Autodesk Fusion 360 part; units mm, degrees
sketch "Esquisse1" plane through (0, 0, 0) normal (0, 0, 1) x (1, 0, 0)
  circle A0 centre (0, 0) radius 12.5
  line L0 (-5.3, -5.3) -> (5.3, -5.3)
  line L1 (5.3, -5.3) -> (5.3, 5.3)
  line L2 (5.3, 5.3) -> (-5.3, 5.3)
  line L3 (-5.3, 5.3) -> (-5.3, -5.3)
  dimension "d1" = 25
  dimension "d4" = 10.6
  dimension "d5" = 5.3
  dimension "d6" = 5.3
extrude "Extrusion1" add sketch "Esquisse1" along normal blind 22 contours A0 | L0 L1 L2 L3
extrude "Extrusion2" cut sketch "Esquisse1" along normal blind 6 contours L0 L1 L2 L3
sketch "Esquisse2" plane through (0, 0, 22) normal (0, 0, 1) x (-1, 0, 0)
  circle A0 centre (0, 0) radius 12.5
  circle A1 centre (0, 0) radius 1.5
  dimension "d9" = 3
extrude "Extrusion3" cut sketch "Esquisse2" against normal blind 22 contours A1
hole "Perçage2" at (0, 0, 6) direction (0, 0, 1) diameter 8 depth 10 tip angle 180
fillet "Congé1" radius 10 1 edges at (-11.6541, -4.5202, 22)
chamfer "Chanfrein1" distance 0.5 angle 45 4 edges at (-5.3, 0, 0) (0, -5.3, 0) (5.3, 0, 0) (0, 5.3, 0)
equation "d5 = d4 / 2"
equation "d6 = d5"
Could you check a few things on this model? Use its own coordinates, in mm. A direction names the side the tool comes from. Coordinates: 2 decimals unless noted, no trailing zeros. Loops run counter-clockwise (first coordinate to the right, second up) from the corner with the lowest first, then second, coordinate; pieces in that order, holes last.
1. Imagine slicing it at B-B (z = 10.25). Please give me the cut outline in (x, y), and give its area (3 significant figures).
2. Imagine slicing it at A-A (z = 2.25). Please give me the cut outline in (x, y).
3. We'd pull the mould along X, two halves only. Please class faces 1 (the face through (0, -8, 0)), 2 (the face through (0, -5.3, 3)), 3 (the face through (11.923, -3.755, 5.916)): released by +X, released by -X, zero draft, split by the parting line, or undercut.
4. For P1, Ø6, axis at y = -6.5, z = 12, coming from the +X side; P2, Ø4, axis at x = -2, y = 3.5, coming from the +Z side; P3, Ø6, axis at x = 2, z = 19.5, coming from the -Y side; P4, Ø4, axis at x = 0, y = 0, coming from the -Z side, each with a flat end and sliding along its axis, tell me the tip position at first contact or that it passes through.
5. I need wall thicknesses on L1, parallel to Y at x = 0, z = 11.5; L2, parallel to Z at x = -1.75, y = 0.25; L3, parallel to X at y = 0, z = 18. Which ranges of each line are inside material? Lowest first, please.
6. For faces 4 (the face through (2, 0, 22)), 5 (the face through (-5.3, 0, 3)), which set-ups out of +Z, -Z, +X, -X, +Y, -Y let a thin tool reach every point of the face, with its end or its side?
Computed values:
1. outline: circle Ø25 at (0, 0); hole circle Ø8 at (0, 0)
1. area: 441 mm2
2. outline: circle Ø25 at (0, 0); hole (-5.3, -5.3) - (5.3, -5.3) - (5.3, 5.3) - (-5.3, 5.3) - close
3. face 1: zero draft
3. face 2: undercut
3. face 3: split by the parting line
4. P1: stops at x = 12
4. P2: stops at z = 22
4. P3: stops at y = -11.31
4. P4: stops at z = 16
5. L1: y = -12.5 to -4, 4 to 12.5
5. L2: z = 16 to 22
5. L3: x = -10.5 to -1.5, 1.5 to 10.5
6. face 4: +Z, +X, -X, +Y, -Y
6. face 5: -Z
